Check sheet for the modelled part. Datum: model origin and axes. Units: mm. A direction names the side the tool comes from. Give positions to 0.01 mm unless a question says otherwise; leave off trailing zeros. Order: outer loops, then holes, each group sorted by start corner. A loop starts at its lowest first (then second) coordinate and runs counter-clockwise, first axis right, second up.
Autodesk Fusion 360 part; units mm, degrees
sketch "Sketch1" plane through (0, 0, 0) normal (0, 1, 0) x (1, 0, 0) in component "Lid"
  line L0 (44.196, 63.5) -> (-44.196, 63.5)
  line L1 (-44.196, 63.5) -> (-44.196, -63.5)
  line L2 (-44.196, -63.5) -> (44.196, -63.5)
  line L3 (44.196, -63.5) -> (44.196, 63.5)
  line L4 (44.196, 63.5) -> (-44.196, -63.5) construction
  line L5 (-44.196, 63.5) -> (44.196, -63.5) construction
  dimension "d1" = 88.392
  dimension "d2" = 127
extrude "Extrude1" add sketch "Sketch1" along normal blind 5.08 in component "Lid"
sketch "Sketch3" plane through (0, 5.08, 0) normal (0, 1, 0) x (-1, 0, 0) in component "Lid"
  line L0 (-44.196, 63.5) -> (-44.196, -63.5)
  line L1 (-44.196, -63.5) -> (44.196, -63.5)
  line L2 (44.196, -63.5) -> (44.196, 63.5)
  line L3 (44.196, 63.5) -> (-44.196, 63.5)
  line L4 (-40.894, -60.198) -> (40.894, -60.198)
  line L5 (40.894, -60.198) -> (40.894, 60.198)
  line L6 (40.894, 60.198) -> (-40.894, 60.198)
  line L7 (-40.894, 60.198) -> (-40.894, -60.198)
  line L8 (-40.894, -60.198) -> (40.894, 60.198) construction
  line L9 (40.894, -60.198) -> (-40.894, 60.198) construction
  dimension "d6" = 81.788
  dimension "d7" = 120.396
extrude "Extrude2" add sketch "Sketch3" along normal blind 5.08 contours L4 L5 L6 L7 in component "Lid"
fillet "Fillet1" radius 2.54 4 edges at (-40.894, 7.62, -60.198) (40.894, 7.62, -60.198) (40.894, 7.62, 60.198) (-40.894, 7.62, 60.198) in component "Lid"
component "Lid" placed x (1, 0, 0) y (0, 1, 0) z (0, 0, 1) at (0, 0, 0)
Q1. Sectioned sample at A-A, the plane z = 30.5. Record the cut outline in (x, y).
Q2. Sectioned sample at B-B, the plane x = -29.5. Record the cut outline in (y, z).
Q3. Material ranges on line 1 (Z direction, x = -4.5, y = 7.75); line 2 (X direction, y = 8.5, z = -20), recorded low to high.
Q4. Go/stop test with flat-tipped pins: P1, Ø5.5, axis at x = 0.5, y = 8.5, coming from the -Z side; P2, Ø1.5, axis at y = 7.5, z = 20, coming from the +X side; P3, Ø4, axis at x = -14.5, y = 8.5, coming from the +Z side. Record where each tip stops, or that it passes through.
Q5. Tool access check on faces 1 (the flat face through (-1, 8, 60.198)), 2 (the flat face through (-40.894, 8, -1)), 3 (the flat face through (40.894, 8, 1)). Record the directions out of +Z, -Z, +X, -X, +Y, -Y that give a thin tool (end or side, any length) a straight path to the whole face; none if there is none.
Filled in:
1. outline: (-44.2, 0) - (44.2, 0) - (44.2, 5.08) - (40.89, 5.08) - (40.89, 10.16) - (-40.89, 10.16) - (-40.89, 5.08) - (-44.2, 5.08) - close
2. outline: (0, -63.5) - (5.08, -63.5) - (5.08, -60.2) - (10.16, -60.2) - (10.16, 60.2) - (5.08, 60.2) - (5.08, 63.5) - (0, 63.5) - close
3. line 1: z = -60.2 to 60.2
3. line 2: x = -40.89 to 40.89
4. P1: stops at z = -60.2
4. P2: stops at x = 40.89
4. P3: stops at z = 60.2
5. face 1: +Z, +X, -X, +Y
5. face 2: +Z, -Z, -X, +Y
5. face 3: +Z, -Z, +X, +Y
